Model file for the job. Use its own axes, mm. A direction names the side the tool comes from. Round coordinates to 2 decimals unless told otherwise and drop trailing zeros. Loops run counter-clockwise (first coordinate to the right, second up) from the corner with the lowest first, then second, coordinate; pieces in that order, holes last. Notation, with made-up numbers: (6.25, 82) -> (47.25, 82) arc R13 ccw to (47.25, 96) -> close; hole circle Ø8 at (-14, -23.5). An arc over 180 degrees is marked (long way). Use a Markdown table: item, result. Add a question column.
```python
from build123d import *

# Parameters (mm, degrees)
F1_R     = 5.715
F1_R_2   = 3.175
F3_R     = 5.715
F3_R_2   = 4.70576
F4_DEPTH = 7


with BuildPart() as f2:
    # F2: sweep along a path in F0
    with BuildLine(Plane.XY) as f2_path:
        ThreePointArc((0, 25), (25, 0), (0, -25))
    # F1 (on Right) → F2 (sweep)
    with BuildSketch(Plane.YZ):
        with Locations((25, 0)):
            Circle(F1_R)
        with Locations((25, 0)):
            Circle(F1_R_2, mode=Mode.SUBTRACT)
    sweep(path=f2_path.line)

    # F3 (on face) → F4 (join)
    with BuildSketch(Plane(origin=(0, 0, 0), x_dir=(0, -1, 0), z_dir=(-1, 0, 0))):
        with Locations((25, 0)):
            Circle(F3_R)
        with Locations((25, 0)):
            Circle(F3_R_2, mode=Mode.SUBTRACT)
        with Locations((-25, 0)):
            Circle(F3_R)
        with Locations((-25, 0)):
            Circle(F3_R_2, mode=Mode.SUBTRACT)
    extrude(amount=F4_DEPTH)


solid = f2.part
```
1) Cut at C-C on x = 15. Count the separate pieces of the cut face and the enclosed holes in it, and give its area (3 significant figures).
2) Wall check: probe 1 along Z at (x, y) = (-1.25, 25) (3 decimals); probe 2 along Y at (x, z) = (7, 2); probe 3 along Y at (x, z) = (-3.5, -4). Give the ranges that are in metal, low to high. Write a range as from..to.
3) Cut at B-B on z = 0. Write the cut outline in (x, y) (3 decimals), and give its area (3 significant figures).
4) Pull direction Z, two halves, no side cores. Call faces 1 (the face through (-3.45, 30.71, 0.25)), 2 (the face through (-3.5, -20.3, 0.2)), 3 (the face through (-7, 24, 5)): +Z half, -Z half, draft (parallel to the pull), parting line (faces both ways), or undercut.
5) Cut at A-A on x = -2.5. Write the cut outline in (y, z) (3 decimals), and give its area (3 significant figures).
6) Tool access for faces 4 (the face through (-7, -26, 5)), 5 (the face through (-3.5, 29.7, 0.2)): list every direction of +Z, -Z, +X, -X, +Y, -Y with a clear straight run to the whole face (end or side of a thin tool).
7) Pin check, flat tips, straight feed: pin 1 Ø1.5 at (y, z) = (-6.5, -1) entering from -X; pin 2 Ø4.5 at (y, z) = (-25, 1.5) entering from -X; pin 3 Ø6 at (y, z) = (15.5, 4.5) entering from -X. Stop position of each tip, or through.
Established:
| question | item | result |
|---|---|---|
| 1 | separate pieces | 2 |
| 1 | enclosed holes | 2 |
| 1 | area | 182 mm^2 |
| 2 | probe 1 | z = -5.715..-4.706, 4.706..5.715 |
| 2 | probe 2 | y = -29.54..-26.56, -21.42..-18.36, 18.36..21.42, 26.56..29.54 |
| 2 | probe 3 | y = -29.08..-27.48, -22.52..-20.92, 20.92..22.52, 27.48..29.08 |
| 3 | outline | (-7, -30.715) -> (0, -30.715) arc R30.715 ccw to (0, 30.715) -> (-7, 30.715) -> (-7, 29.706) -> (0, 29.706) -> (0, 28.175) arc R28.175 cw to (0, -28.175) -> (0, -29.706) -> (-7, -29.706) -> close; (-7, -20.294) -> (0, -20.294) -> (0, -21.825) arc R21.825 ccw to (0, 21.825) -> (0, 20.294) -> (-7, 20.294) -> (-7, 19.285) -> (0, 19.285) arc R19.285 cw to (0, -19.285) -> (-7, -19.285) -> close |
| 3 | area | 427 mm^2 |
| 4 | face 1 | parting line |
| 4 | face 2 | undercut |
| 4 | face 3 | draft |
| 5 | outline | circle Ø11.43 at (-25, 0); circle Ø11.43 at (25, 0); hole circle Ø9.412 at (-25, 0); hole circle Ø9.412 at (25, 0) |
| 5 | area | 66.1 mm^2 |
| 6 | face 4 | +Z, -Z, -X, +Y, -Y |
| 6 | face 5 | -X |
| 7 | pin 1 | stops at x = 17.94 |
| 7 | pin 2 | stops at x = 0 |
| 7 | pin 3 | stops at x = 8.81 |
